Autodesk Inventor part; units mm, degrees
ref_plane "YZ Plane" through (0, 0, 0) normal (1, 0, 0) x (0, 1, 0)
ref_plane "XZ Plane" through (0, 0, 0) normal (0, 1, 0) x (-1, 0, 0)
ref_plane "XY Plane" through (0, 0, 0) normal (0, 0, 1) x (1, 0, 0)
sketch "Sketch1" plane through (0, 0, 0) normal (0, 0, 1) x (1, 0, 0)
  line L0 (0, 0) -> (50.8, 0)
  line L1 (50.8, 0) -> (50.8, 50.8)
  line L2 (50.8, 50.8) -> (0, 50.8)
  line L3 (0, 50.8) -> (0, 0)
  line L4 (3.175, 3.175) -> (47.625, 3.175)
  line L5 (47.625, 3.175) -> (47.625, 47.625)
  line L6 (47.625, 47.625) -> (3.175, 47.625)
  line L7 (3.175, 47.625) -> (3.175, 3.175)
  dimension "d0" = 50.8
  dimension "d1" = 50.8
  dimension "d2" = 3.175
  dimension "d3" = 3.175
  dimension "d4" = 3.175
  dimension "d5" = 3.175
extrude "2x2x.125 Box Beam" add sketch "Sketch1" along normal blind 127
sketch "Sketch2" plane through (50.8, 0, 0) normal (1, 0, 0) x (0, 0, -1)
  line L0 (0, 0) -> (0, 50.8)
  line L1 (0, 0) -> (-127, 0)
  circle A0 centre (-63.5, 25.4) radius 14.2875
  dimension "d8" = 28.575
  dimension "d9" = 63.5
  dimension "d10" = 25.4
extrude "FR8 Bearing Hole" cut sketch "Sketch2" against normal through all
equation "\"d3\" = d2"
equation "\"d4\" = d3"
equation "\"d5\" = d4"
properties part number "Box Beam"
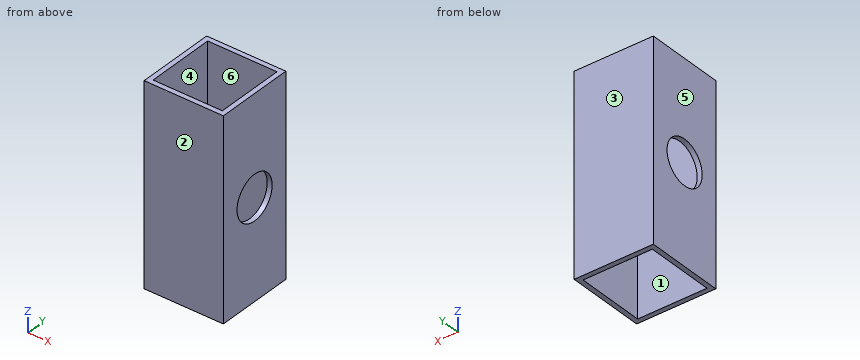
Check sheet for the modelled part. Datum: model origin and axes. Units: mm. Face numbers are marked on the shaded views. A direction names the side the tool comes from. Round coordinates to 2 decimals unless told otherwise and drop trailing zeros. Write each loop counter-clockwise with the first axis right and the second up, starting at its lowest first coordinate (ties: lowest second). Pieces come first, ordered by that corner, then holes. Notation, with made-up numbers: (10.25, 85) - (18.25, 85) arc R16 ccw to (18.25, 98) - close; hole circle Ø1 at (52.5, 83). An arc over 180 degrees is marked (long way). Return JSON: item names as keys, results as strings.
Q1. Scan lines: L1, parallel to X at y = 12, z = 52.5 (3 decimals); L2, parallel to Y at x = 2.3, z = 63.5. Record each from-to range of solid material in increasing order. Write a range as from..to.
Returned:
{"L1": "x = 0..3.175, 47.625..50.8", "L2": "y = 0..11.11, 39.69..50.8"}
Q2. Access from +Z, -Z, +X, -X, +Y, -Y to the whole of each face (thin tool, end or side, straight path). Record for the marked faces 1 and 2.
Returned:
{"face 1": "+Z, -Z", "face 2": "+Z, -Z, +X, -X, -Y"}
Q3. Draft check along X on the marked faces 3, 4, 5 and 6. Enter one of: released by +X, released by -X, zero draft, split by the parting line, or undercut.
Returned:
{"face 3": "zero draft", "face 4": "undercut", "face 5": "released by -X", "face 6": "undercut"}
Q4. Depth check by flat-ended pin: P1, Ø13.5, axis at x = 28.5, z = 62, coming from the -Y side. Enter the tip coordinate at first touch or a pass-through.
Returned:
{"P1": "stops at y = 0"}
Q5. Cross-section at D-D (y = 22). Record the boundary of the cut face in (x, z) (3 decimals).
Returned:
{"outline": "(0, 0) - (3.175, 0) - (3.175, 49.623) - (0, 49.623) - close; (0, 77.377) - (3.175, 77.377) - (3.175, 127) - (0, 127) - close; (47.625, 0) - (50.8, 0) - (50.8, 49.623) - (47.625, 49.623) - close; (47.625, 77.377) - (50.8, 77.377) - (50.8, 127) - (47.625, 127) - close"}
Q6. Cross-section at A-A (y = 45.5). Record the boundary of the cut face in (x, z) (3 decimals).
Returned:
{"outline": "(0, 0) - (3.175, 0) - (3.175, 127) - (0, 127) - close; (47.625, 0) - (50.8, 0) - (50.8, 127) - (47.625, 127) - close"}
Q7. Cross-section at B-B (z = 63.5). Record the boundary of the cut face in (x, y) (1 decimal), then the cut area to 3 significant figures.
Returned:
{"outline": "(0, 0) - (50.8, 0) - (50.8, 11.1) - (47.6, 11.1) - (47.6, 3.2) - (3.2, 3.2) - (3.2, 11.1) - (0, 11.1) - close; (0, 39.7) - (3.2, 39.7) - (3.2, 47.6) - (47.6, 47.6) - (47.6, 39.7) - (50.8, 39.7) - (50.8, 50.8) - (0, 50.8) - close", "area": "423 mm²"}
